Part model, mm, in its own coordinate system. A direction names the side the tool comes from. Coordinates: 2 decimals unless noted, no trailing zeros. Write each loop counter-clockwise with the first axis right and the second up, starting at its lowest first coordinate (ties: lowest second). Pieces come first, ordered by that corner, then holes. Notation, with made-up numbers: (-27.75, 23.5) -> (-7.75, 23.5) arc R17 ccw to (-7.75, 43.5) -> close; hole circle Ø6 at (73, 10). An arc over 180 degrees is marked (long way). Write item = value, one per line.
from build123d import *

# Parameters (mm, degrees)
SKETCH1_W           = 442
SKETCH1_H           = 420
BOSS_EXTRUDE1_DEPTH = 2
SKETCH2_W           = 1
SKETCH2_H           = 408
BOSS_EXTRUDE2_DEPTH = 10
FILLET1_R           = 2
FILLET2_R           = 0.5
FILLET3_R           = 1
FILLET4_R           = 0.5


with BuildPart() as part:
    # Sketch1 → Boss-Extrude1 (new body)
    with BuildSketch(Plane(origin=(0, 0, 0), x_dir=(1, 0, 0), z_dir=(0, 1, 0))):
        Rectangle(SKETCH1_W, SKETCH1_H)
    extrude(amount=BOSS_EXTRUDE1_DEPTH)

    # Sketch2 → Boss-Extrude2 (add)
    with BuildSketch(Plane.XZ):
        with Locations((220.5, 6)):
            Rectangle(SKETCH2_W, SKETCH2_H)
        with Locations((-220.5, 6)):
            Rectangle(SKETCH2_W, SKETCH2_H)
    extrude(amount=BOSS_EXTRUDE2_DEPTH)

    # Fillet1
    fillet1_edges = [part.edges().sort_by_distance(p)[0] for p in [
        (-220.5, -10, -198),
        (220.5, -10, -198),
    ]]
    fillet(fillet1_edges, radius=FILLET1_R)

    # Fillet2
    fillet2_edges = [part.edges().sort_by_distance(p)[0] for p in [
        (-220.5, 0, -198),
        (220.5, 0, -198),
    ]]
    fillet(fillet2_edges, radius=FILLET2_R)

    # Fillet3
    fillet3_edges = [part.edges().sort_by_distance(p)[0] for p in [
        (-221, 2, 0),
        (221, 2, 0),
    ]]
    fillet(fillet3_edges, radius=FILLET3_R)

    # Fillet4
    fillet4_edges = [part.edges().sort_by_distance(p)[0] for p in [
        (-220, 0, 5.75),
        (220, 0, 5.75),
    ]]
    fillet(fillet4_edges, radius=FILLET4_R)


solid = part.part
Q1. Saw through at B-B on z = -148. Give the cut face in (x, y), and give its area (3 significant figures).
Model answer:
outline = (-221, -10) -> (-220, -10) -> (-220, -0.5) arc R0.5 cw to (-219.5, 0) -> (219.5, 0) arc R0.5 cw to (220, -0.5) -> (220, -10) -> (221, -10) -> (221, 1) arc R1 ccw to (220, 2) -> (-220, 2) arc R1 ccw to (-221, 1) -> close
area = 904 mm²
Q2. Mould opens along X. For faces 3 (the face through (221, -4, -3)), 4 (the face through (220, -5, 3)), 5 (the face through (-1, 1, 210)) say: released by +X, released by -X, zero draft, split by the parting line, or undercut.
Model answer:
face_3 = released by +X
face_4 = undercut
face_5 = zero draft
Q3. Saw through at A-A on y = -2.75. Give the cut face in (x, z).
Model answer:
outline = (-221, -198) -> (-220, -198) -> (-220, 210) -> (-221, 210) -> close; (220, -198) -> (221, -198) -> (221, 210) -> (220, 210) -> close
Q4. Saw through at C-C on x = 57. Give the cut face in (y, z).
Model answer:
outline = (0, -210) -> (2, -210) -> (2, 210) -> (0, 210) -> close
Q5. Probe line 1 (X direction, y = -1.25, z = -26); line 2 (Y direction, x = 35, z = 155.5); line 3 (X direction, y = -0.25, z = -48.5). List the from-to ranges inside material, lowest first. Write a range as from..to.
Model answer:
line_1 = -221..-220, 220..221
line_2 = 0..2
line_3 = -221..-219.93, 219.93..221
Q6. Pin check, flat tips, straight feed: pin 1 (0.5 mm diameter, centred on x = 220.5, y = -5.5, fed in from -Z); pin 2 (4 mm diameter, centred on x = 14, z = 154, fed in from -Y). Stop position of each tip, or through.
Model answer:
pin_1 = -198
pin_2 = 0
Q7. Which spindle directions (+Z, -Z, +X, -X, +Y, -Y) get a long thin tool onto all of the face, cutting with end or side? Do faces 1 (the face through (-3, 0, -3)), 2 (the face through (-221, -5, 3)). Say none if no direction does.
Model answer:
face_1 = +Z, -Z, -Y
face_2 = +Z, -Z, -X, +Y, -Y
